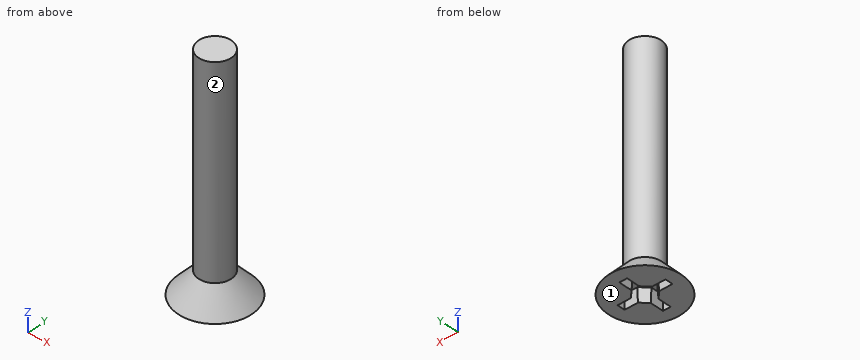
```python
from build123d import *

# Parameters (mm, degrees)
H1_CROSSRECESS_4DEG_DEPTH = 0.762
H1_CROSSRECESS_4DEG_DRAFT = 4


with BuildPart() as part:
    # H1_SK_profile → H1_Body (revolve)
    with BuildSketch(Plane(origin=(0, 0, 0), x_dir=(0, 0, -1), z_dir=(1, 0, 0)), mode=Mode.PRIVATE) as h1_body_sk:
        Polygon((11.43, 0), (11.43, 2.0574), (10.16, 0.9144), (-1.27, 0.9144), (-1.27, 0), align=None)
    revolve(h1_body_sk.sketch.rotate(Axis((0, 0, -15.24), (0, 0, 1)), 90), axis=Axis((0, 0, -15.24), (0, 0, 1)))


with BuildPart() as h1_crossrecess_4deg_tool:
    # H1_SK_crossRecess → H1_CrossRecess_4deg (with draft: the straight prism first)
    with BuildSketch(Plane.XY.offset(-11.43)):
        Polygon((1.3462, -0.2159), (1.3462, 0.2159), (0.5969, 0.2159), (0.2159, 0.5969), (0.2159, 1.3462), (-0.2159, 1.3462), (-0.2159, 0.5969), (-0.5969, 0.2159), (-1.3462, 0.2159), (-1.3462, -0.2159), (-0.5969, -0.2159), (-0.2159, -0.5969), (-0.2159, -1.3462), (0.2159, -1.3462), (0.2159, -0.5969), (0.5969, -0.2159), align=None)
    extrude(amount=H1_CROSSRECESS_4DEG_DEPTH)
    # H1_CrossRecess_4deg: the draft: its side faces are tilted about the plane it starts from
    h1_crossrecess_4deg_sides = [h1_crossrecess_4deg_tool.faces().sort_by_distance(p)[0] for p in [
        (1.3462, 0, -11.049),
        (0.97155, 0.2159, -11.049),
        (0.4064, 0.4064, -11.049),
        (0.2159, 0.97155, -11.049),
        (0, 1.3462, -11.049),
        (-0.2159, 0.97155, -11.049),
        (-0.4064, 0.4064, -11.049),
        (-0.97155, 0.2159, -11.049),
        (-1.3462, 0, -11.049),
        (-0.97155, -0.2159, -11.049),
        (-0.4064, -0.4064, -11.049),
        (-0.2159, -0.97155, -11.049),
        (0, -1.3462, -11.049),
        (0.2159, -0.97155, -11.049),
        (0.4064, -0.4064, -11.049),
        (0.97155, -0.2159, -11.049),
    ]]
    draft(h1_crossrecess_4deg_sides, Plane.XY.offset(-11.43), H1_CROSSRECESS_4DEG_DRAFT)


with BuildPart() as part_1:
    add(part.part)

    # H1_CrossRecess_4deg: cut by h1_crossrecess_4deg_tool
    add(h1_crossrecess_4deg_tool.part, mode=Mode.SUBTRACT)


solid = part_1.part
```
Could you check a few things on this model? Use its own coordinates, in mm. Face numbers are marked on the shaded views. A direction names the side the tool comes from. Round coordinates to 2 decimals unless told otherwise and drop trailing zeros. Loops run counter-clockwise (first coordinate to the right, second up) from the corner with the lowest first, then second, coordinate; pieces in that order, holes last. Notation, with made-up numbers: M 36.25,5 L 92.25,5 A13 ccw 92.25,29 Z; hole C -17,41 d8. An arc over 180 degrees is marked long. Write item = value, one per line.
1. I need wall thicknesses on probe 1 along Z at (x, y) = (-0.1, 0.2); probe 2 along Y at (x, z) = (0, -4.75); probe 3 along X at (y, z) = (-0.75, -5.25). Which ranges of each line are inside material? Lowest first, please.
Results below:
probe_1 = -10.67 to 1.27
probe_2 = -0.91 to 0.91
probe_3 = -0.52 to 0.52
2. I want a section at C-C, the plane z = 0. Write out the boundary of the cut face in (x, y), and give its area (3 significant figures).
Results below:
outline = C 0,0 d1.83
area = 2.63 mm²
3. I want a section at A-A, the plane y = 0. Write out the boundary of the cut face in (x, z), and give its area (3 significant figures).
Results below:
outline = M -2.06,-11.43 L -1.35,-11.43 L -1.29,-10.67 L 1.29,-10.67 L 1.35,-11.43 L 2.06,-11.43 L 0.91,-10.16 L 0.91,1.27 L -0.91,1.27 L -0.91,-10.16 Z
area = 22.7 mm²
4. Which directions (+Z, -Z, +X, -X, +Y, -Y) give clear straight access to the entire face, cutting with the end or side of a thin tool? Please do the marked faces 1 and 2.
Results below:
face_1 = -Z, +X, -X, +Y, -Y
face_2 = +Z
